from build123d import *

# Parameters (mm, degrees)
ESQUISSE1_R        = 51.1
BOSS_EXTRU_1_DEPTH = 11.482
SKETCH2_R          = 1.6
CUT_EXTRUDE1_DEPTH = 107.685689406
CIRPATTERN1_COUNT  = 9
SKETCH3_R          = 2.2
CUT_EXTRUDE2_DEPTH = 25
CIRPATTERN2_COUNT  = 12


with BuildPart() as part:
    # Esquisse1 → Boss.-Extru.1 (new body)
    with BuildSketch(Plane.XY):
        with BuildLine():
            Line((52.641728383, -37.021851843), (61.890836376, -42.361826833))
            ThreePointArc((61.890836376, -42.361826833), (0, -75), (-61.890836376, -42.361826833))
            Line((-61.890836376, -42.361826833), (-52.641728383, -37.021851843))
            Line((-52.641728383, -37.021851843), (-58.382728383, -27.078148157))
            Line((-58.382728383, -27.078148157), (-67.631836376, -32.418123147))
            ThreePointArc((-67.631836376, -32.418123147), (-64.951905284, 37.5), (-5.741, 74.77994998))
            Line((-5.741, 74.77994998), (-5.741, 64.1))
            Line((-5.741, 64.1), (5.741, 64.1))
            Line((5.741, 64.1), (5.741, 74.77994998))
            ThreePointArc((5.741, 74.77994998), (64.951905284, 37.5), (67.631836376, -32.418123147))
            Line((67.631836376, -32.418123147), (58.382728383, -27.078148157))
            Line((58.382728383, -27.078148157), (52.641728383, -37.021851843))
        make_face()
        Circle(ESQUISSE1_R, mode=Mode.SUBTRACT)
    extrude(amount=BOSS_EXTRU_1_DEPTH)

    # Sketch2 → Cut-Extrude1 (cut, through all)
    with BuildSketch(Plane.XY.offset(11.482)):
        with Locations((22.573329459, 62.019712972)):
            Circle(SKETCH2_R)
    cut_extrude1 = extrude(amount=-CUT_EXTRUDE1_DEPTH, mode=Mode.SUBTRACT)

    # CirPattern1: Cut-Extrude1 ×9 about axis
    cirpattern1_axis = Axis((0, 0, 0), (0, 0, 1))
    for i in range(1, CIRPATTERN1_COUNT):
        add(cut_extrude1.rotate(cirpattern1_axis, i * 360 / CIRPATTERN1_COUNT), mode=Mode.SUBTRACT)

    # Sketch3 → Cut-Extrude2 (cut, symmetric)
    with BuildSketch(Plane.XY):
        with Locations((15.316911089, 57.1634904)):
            Circle(SKETCH3_R)
    cut_extrude2 = extrude(amount=CUT_EXTRUDE2_DEPTH, both=True, mode=Mode.SUBTRACT)

    # CirPattern2: Cut-Extrude2 ×12 about axis
    cirpattern2_axis = Axis((0, 0, 0), (0, 0, 1))
    for i in range(1, CIRPATTERN2_COUNT):
        add(cut_extrude2.rotate(cirpattern2_axis, i * 360 / CIRPATTERN2_COUNT), mode=Mode.SUBTRACT)


solid = part.part
The listing builds one solid part. Answer for the finished solid, in the listing's coordinates (mm). A direction names the side the tool comes from. Round coordinates to 2 decimals unless told otherwise and drop trailing zeros. Write each loop counter-clockwise with the first axis right and the second up, starting at its lowest first coordinate (ties: lowest second). Pieces come first, ordered by that corner, then holes. Notation, with made-up numbers: (79.5, 14) - (108.5, 14) arc R30 cw to (108.5, 42) - close; hole circle Ø4 at (59, -28.75). An arc over 180 degrees is marked (long way). Use a Markdown table: item, result. Add a question column.
1. The part is cut by section B-B (x = 10). Write down the section's boundary in (y, z).
2. The part is cut by section C-C (z = 4.5). Give the number of separate pieces and of enclosed holes in the cut face, and give its area (3 significant figures).
3. A tool of negligible diameter and unlimited length cuts with its end or side. For faces 1 (the face through (64.436, 38.379, 5.661)), 2 (the face through (63.1, -29.8, 5.7)), 3 (the face through (5.741, 69, 6)), from which of +Z, -Z, +X, -X, +Y, -Y can it reach the whole face along a straight path? Write none if from no direction.
4. Flat-ended cylindrical pins translate along their axes: P1, Ø5.5, axis at x = 2.5, z = 5.5, coming from the +Y side; P2, Ø3, axis at y = 55.5, z = 2, coming from the +X side; P3, Ø1, axis at x = -21.5, z = 5.5, coming from the +Y side. Find the tip coordinate at first contact, or state that the pin passes through.
5. Consider line 1 (Y direction, x = 23, z = 2); line 2 (Y direction, x = -17, z = 1.5); line 3 (Y direction, x = -42, z = 2.75). Determine where each line is inside the solid, lowest interval first.
6. For a pull along X with two mould halves and no side action, classify faces 4 (the face through (-49, -16, 11.482)), 5 (the face through (57.202, -39.654, 5.661)), 6 (the face through (-42.69, -43.88, 5.82)) as +X half, -X half, draft (parallel to the pull), parting line (faces both ways), or undercut.
7. The part is cut by section A-A (y = 0). Write down the section's boundary in (x, z), and give its area (3 significant figures).
Reported:
| question | item | result |
|---|---|---|
| 1 | outline | (-74.33, 0) - (-50.11, 0) - (-50.11, 11.48) - (-74.33, 11.48) - close; (50.11, 0) - (74.33, 0) - (74.33, 11.48) - (50.11, 11.48) - close |
| 2 | separate pieces | 1 |
| 2 | enclosed holes | 22 |
| 2 | area | 8,840 mm^2 |
| 3 | face 1 | +Z, -Z, +X |
| 3 | face 2 | +Z, -Z |
| 3 | face 3 | +Z, -Z, +Y |
| 4 | P1 | y = 64.1 |
| 4 | P2 | x = 52.05 |
| 4 | P3 | y = 72 |
| 5 | line 1 | -71.39 to -45.63, 45.63 to 60.48, 63.56 to 71.39 |
| 5 | line 2 | -73.05 to -58.58, -55.75 to -48.19, 48.19 to 55.75, 58.58 to 73.05 |
| 5 | line 3 | -62.14 to -52.1, -49.02 to -44.04, -39.65 to -29.11, 29.11 to 39.65, 44.04 to 62.14 |
| 6 | face 4 | draft |
| 6 | face 5 | +X half |
| 6 | face 6 | undercut |
| 7 | outline | (-75, 0) - (-51.1, 0) - (-51.1, 11.48) - (-75, 11.48) - close; (51.1, 0) - (75, 0) - (75, 11.48) - (51.1, 11.48) - close |
| 7 | area | 549 mm^2 |
